Could you check a few things on this drawing? It's one solid part, dimensions in mm from its lowest x, y, z. A direction names the side the tool comes from. Coordinates: 2 decimals unless noted, no trailing zeros. Order: outer loops, then holes, each group sorted by start corner. A loop starts at its lowest first (then second) coordinate and runs counter-clockwise, first axis right, second up. Notation, with made-up numbers: (89.5, -22) -> (126.5, -22) arc R25 cw to (126.5, 13) -> close; hole circle Ø7 at (4, 65.25). An arc over 180 degrees is marked (long way). Use a Markdown table: item, result. Add a question column.
1. If I drill on line 1 along Z through (x, y) = (13.75, 3.75); line 2 along Y through (x, z) = (9, 2.75); line 3 along Z through (x, y) = (14.75, 2.25), over which ranges is the centre line in solid material (lowest first)? Write a range as from..to.
2. For the marked faces 1 and 2, which set-ups out of +Z, -Z, +X, -X, +Y, -Y let a thin tool reach every point of the face, with its end or its side?
3. Suppose I cut it at A-A, the plane x = 13.4. List the corners of the cut face in (y, z) for me.
4. For pin 1 Ø1 at (x, z) = (6, 3.5) entering from +Y; pin 2 Ø1.8 at (x, y) = (17.5, 4.5) entering from -Z, each with a flat end and sliding along its axis, tell me the tip position at first contact or that it passes through.
5. Suppose I cut it at B-B, the plane z = 7. List the corners of the cut face in (x, y) for me, then the cut area to 3 significant figures.
6. We'd pull the mould along X, two halves only. Please class the marked faces 3, 4, 5 and 6: pulls with the +X half, pulls with the -X half, needs draft (parallel to the pull), parting line crosses it, or undercut.
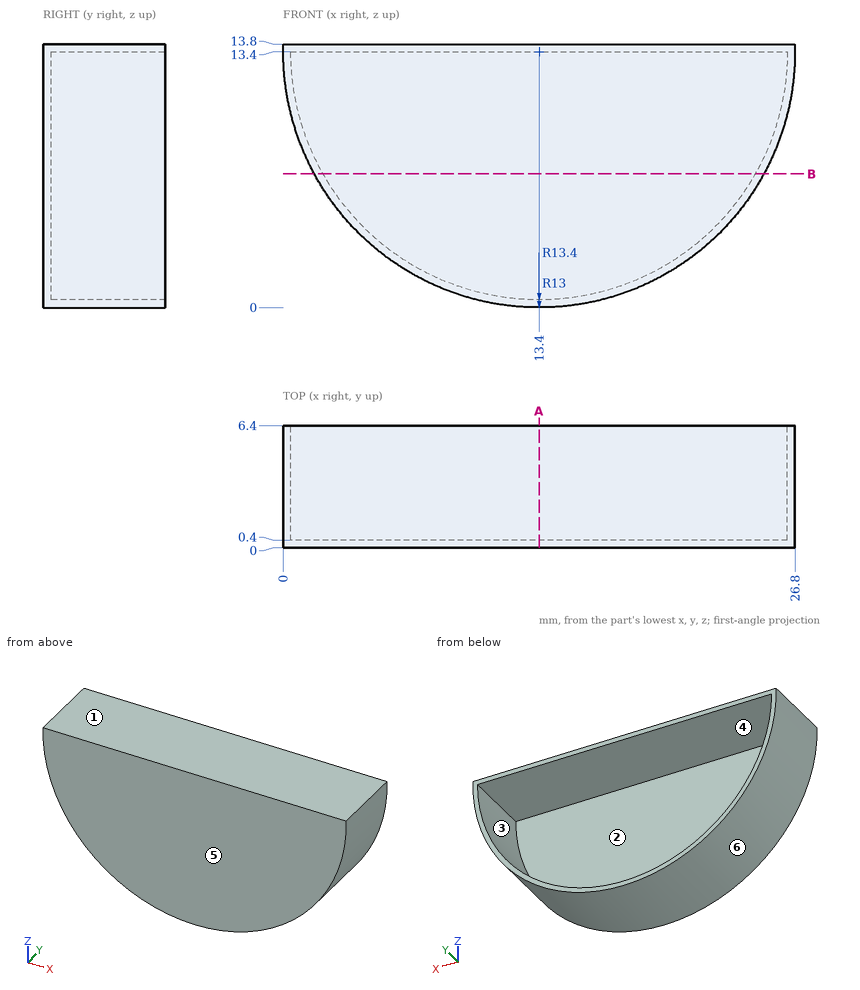
Worked out:
| question | item | result |
|---|---|---|
| 1 | line 1 | z = 0..0.4, 13.4..13.8 |
| 1 | line 2 | y = 0..0.4 |
| 1 | line 3 | z = 0.07..0.47, 13.4..13.8 |
| 2 | face 1 | +Z, +X, -X, +Y, -Y |
| 2 | face 2 | +Y |
| 3 | outline | (0, 0) -> (6.4, 0) -> (6.4, 0.4) -> (0.4, 0.4) -> (0.4, 13.4) -> (6.4, 13.4) -> (6.4, 13.8) -> (0, 13.8) -> close |
| 4 | pin 1 | stops at y = 0.4 |
| 4 | pin 2 | stops at z = 0.39 |
| 5 | outline | (1.63, 0) -> (25.17, 0) -> (25.17, 6.4) -> (24.72, 6.4) -> (24.72, 0.4) -> (2.08, 0.4) -> (2.08, 6.4) -> (1.63, 6.4) -> close |
| 5 | area | 14.9 mm² |
| 6 | face 3 | undercut |
| 6 | face 4 | undercut |
| 6 | face 5 | needs draft |
| 6 | face 6 | parting line crosses it |
